Part print with two shaded views. Sizes in mm from the minimum x, y, z corner. Coordinates: 2 decimals unless noted, no trailing zeros. Loops run counter-clockwise (first coordinate to the right, second up) from the corner with the lowest first, then second, coordinate; pieces in that order, holes last. Notation, with made-up numbers: (-24.5, -21.5) - (33.5, -21.5) arc R28 ccw to (33.5, 5.5) - close; hole circle Ø3 at (34, 73). An arc over 180 degrees is marked (long way). Write each question's results on one line, items separated by ' | '. Start each with the question number.
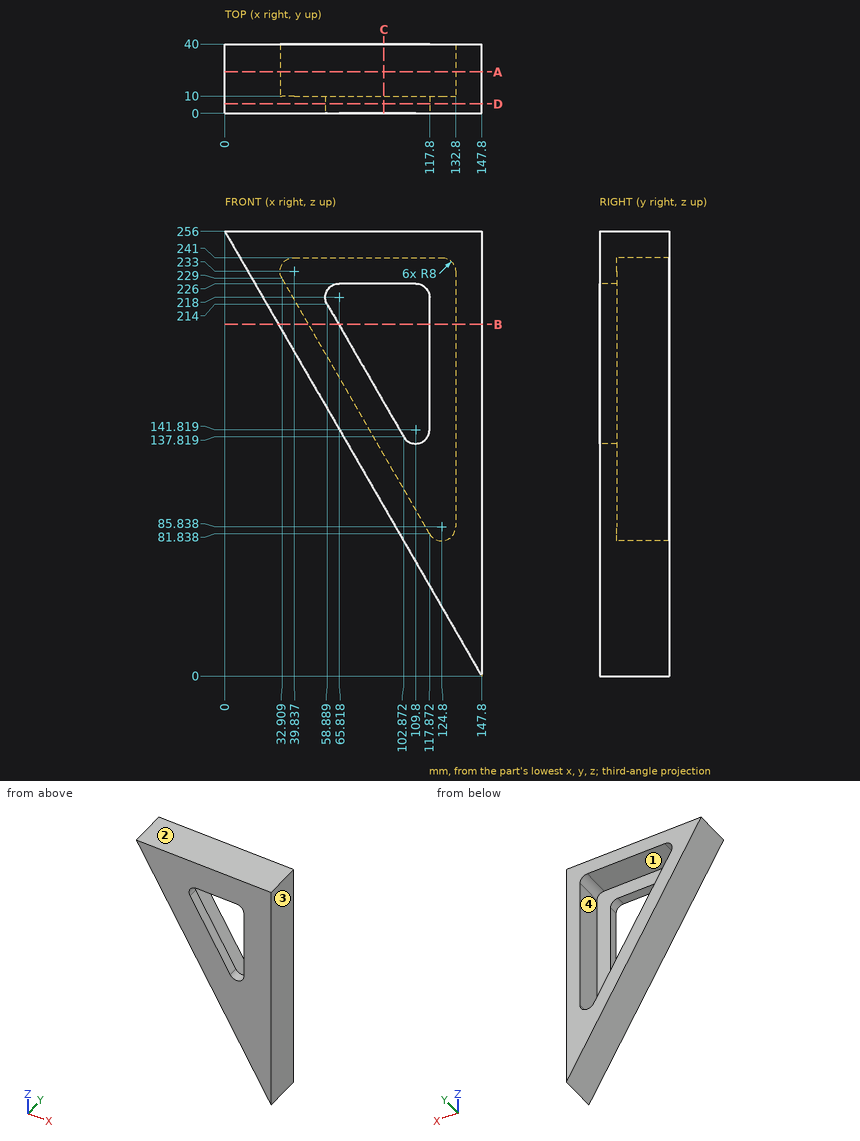
Q1. Drill centre lines: L1, parallel to Z at x = 96, y = 19 (1 decimal); L2, parallel to X at y = 4, z = 185; L3, parallel to Y at x = 131, z = 130. Where is each one in solid material? Low to high. Write a range as from..to.
Q2. Cut at A-A (y = 24). List the corners of the cut face in (x, z), and give its area (3 significant figures).
Q3. Cut at C-C (x = 91.5). List the corners of the cut face in (y, z) (1 decimal).
Q4. Cut at B-B (z = 202.5). List the corners of the cut face in (x, y), and give its area (3 significant figures).
Q5. Mould opens along X. For the marked faces 1, 2, 3 and 4 say: +X half, -X half, draft (parallel to the pull), parting line (faces both ways), or undercut.
Q6. Cut at D-D (y = 5.5). List the corners of the cut face in (x, z).
Q7. Pin check, flat tips, straight feed: pin 1 (15 mm diameter, centred on x = 62.5, y = 26.5, fed in from -Z) (1 decimal); pin 2 (8 mm diameter, centred on x = 79, y = 5, fed in from -Z); pin 3 (8 mm diameter, centred on y = 4, z = 162.5, fed in from -X). Stop position of each tip, or through.
Check result:
1) L1: 89.7..119.7, 241..256 | L2: 40.99..75.63, 117.8..147.8 | L3: 0..10
2) outline: (0, 256) - (147.8, 0) - (147.8, 256) - close; hole (32.91, 229) - (117.87, 81.84) arc R8 ccw to (132.8, 85.84) - (132.8, 233) arc R8 ccw to (124.8, 241) - (39.84, 241) arc R8 ccw to start | area: 9,250 mm²
3) outline: (0, 97.5) - (40, 97.5) - (40, 127.5) - (10, 127.5) - (10, 157.5) - (0, 157.5) - close; (0, 226) - (10, 226) - (10, 241) - (40, 241) - (40, 256) - (0, 256) - close
4) outline: (30.89, 0) - (65.53, 0) - (65.53, 10) - (48.21, 10) - (48.21, 40) - (30.89, 40) - close; (117.8, 0) - (147.8, 0) - (147.8, 40) - (132.8, 40) - (132.8, 10) - (117.8, 10) - close | area: 1,620 mm²
5) face 1: undercut | face 2: draft | face 3: +X half | face 4: undercut
6) outline: (0, 256) - (147.8, 0) - (147.8, 256) - close; hole (58.89, 214) - (102.87, 137.82) arc R8 ccw to (117.8, 141.82) - (117.8, 218) arc R8 ccw to (109.8, 226) - (65.82, 226) arc R8 ccw to start
7) pin 1: z = 134.8 | pin 2: z = 112.24 | pin 3: x = 51.67
